The listing builds one solid part. Answer for the finished solid, in the listing's coordinates (mm). Round coordinates to 2 decimals unless told otherwise and drop trailing zeros. Loops run counter-clockwise (first coordinate to the right, second up) from the corner with the lowest first, then second, coordinate; pieces in that order, holes last. Notation, with made-up numbers: (-14, 68) -> (35, 68) arc R22 cw to (35, 77) -> close; hole circle Ø10 at (44, 8). An arc over 180 degrees is marked (long way). Use a Markdown table: item, result. Add a question column.
Q1. Given pin 1 Ø1 at (x, z) = (-13.73, -10.14) entering from -Y, flat-ended and moving along its own axis, determine where the tip first touches the part or whether it passes through.
Q2. Section A-A on y = 1 is taken. Give the number of separate pieces and of enclosed holes in the cut face, then the cut area to 3 significant figures.
Q3. Section B-B on z = 9 is taken. Give the vertices of the cut face in (x, y) (3 decimals).
Q4. Consider line 1 (Z direction, x = 7, y = 0.8) (3 decimals); line 2 (Z direction, x = 6.5, y = 0.7) (3 decimals). Determine where each line is inside the solid, lowest interval first.
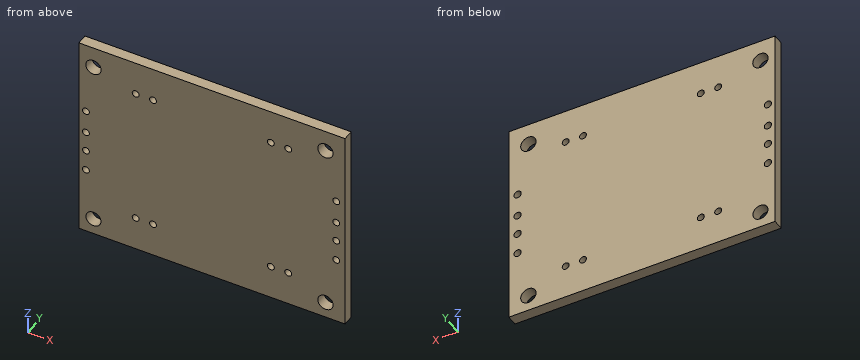
from build123d import *

# Parameters (mm, degrees)
SKETCH_1_W               = 30.85
SKETCH_1_H               = 24.07
EXTRUDE_1_DEPTH          = 1.25
CUT_EXTRUDE_1_DEPTH      = 11
CUT_EXTRUDE_1_DEPTH_BACK = 11
SKETCH_2_R               = 0.872176239
SKETCH_2_R_2             = 0.89
SKETCH_2_R_3             = 0.4


# Read off the part's stored shape, not the designer's step: 切除-拉伸2
with BuildPart() as part:
    # 草图1 → 凸台-拉伸1 (new body)
    with BuildSketch(Plane(origin=(0, 0, 0), x_dir=(1, 0, 0), z_dir=(0, 1, 0))):
        Rectangle(SKETCH_1_W, SKETCH_1_H)
    extrude(amount=EXTRUDE_1_DEPTH)

    # 草图2 → 切除-拉伸1 (cut, two sides: drawn at the far end of the back side and taken through both)
    with BuildSketch(Plane(origin=(0, 0, 0), x_dir=(1, 0, 0), z_dir=(0, 1, 0)).offset(-CUT_EXTRUDE_1_DEPTH_BACK)):
        with Locations(Location((-13.728729398, 10.145, 0), (0, 0, 270))):
            Circle(SKETCH_2_R)
        with Locations(Location((-13.728729398, -9.533026001, 0), (0, 0, 270))):
            Circle(SKETCH_2_R_2)
        with Locations(Location((13.15647485, -9.533026001, 0), (0, 0, 270))):
            Circle(SKETCH_2_R_2)
        with Locations(Location((13.15647485, 10.145, 0), (0, 0, 270))):
            Circle(SKETCH_2_R_2)
        with Locations(Location((-8.835, 8.055, 0), (0, 0, 270))):
            Circle(SKETCH_2_R_3)
        with Locations(Location((-6.825, 8.055, 0), (0, 0, 270))):
            Circle(SKETCH_2_R_3)
        with Locations(Location((6.825, 8.055, 0), (0, 0, 270))):
            Circle(SKETCH_2_R_3)
        with Locations(Location((8.835, 8.055, 0), (0, 0, 270))):
            Circle(SKETCH_2_R_3)
        with Locations(Location((-8.835, -8.055, 0), (0, 0, 270))):
            Circle(SKETCH_2_R_3)
        with Locations(Location((-6.825, -8.055, 0), (0, 0, 270))):
            Circle(SKETCH_2_R_3)
        with Locations(Location((6.825, -8.055, 0), (0, 0, 270))):
            Circle(SKETCH_2_R_3)
        with Locations(Location((8.835, -8.055, 0), (0, 0, 270))):
            Circle(SKETCH_2_R_3)
    extrude(amount=CUT_EXTRUDE_1_DEPTH + CUT_EXTRUDE_1_DEPTH_BACK, mode=Mode.SUBTRACT)

    # 切除-拉伸2 outline → 切除-拉伸2 (revolve, cut)
    with BuildSketch(Plane(origin=(14.403562721, 0, -4.132088396), x_dir=(1, 0, 0), z_dir=(0, 0, 1))):
        Polygon((0.421818831, 1.25), (0, 1.25), (0, 0), (0.4, 0), align=None)
    revolve(axis=Axis((14.403562721, 0, -4.132088396), (0, 1, 0)), mode=Mode.SUBTRACT)

    # Cut-Extrude 2 2 outline → Cut-Extrude 2 2 (revolve, cut)
    with BuildSketch(Plane(origin=(-14.599926989, 0, -4.132088396), x_dir=(1, 0, 0), z_dir=(0, 0, 1))):
        Polygon((0.421818831, 1.25), (0, 1.25), (0, 0), (0.4, 0), align=None)
    revolve(axis=Axis((-14.599926989, 0, -4.132088396), (0, 1, 0)), mode=Mode.SUBTRACT)

    # Cut-Extrude 2 3 outline → Cut-Extrude 2 3 (revolve, cut)
    with BuildSketch(Plane(origin=(14.403562721, 0, -1.635099216), x_dir=(1, 0, 0), z_dir=(0, 0, 1))):
        Polygon((0.421818831, 1.25), (0, 1.25), (0, 0), (0.4, 0), align=None)
    revolve(axis=Axis((14.403562721, 0, -1.635099216), (0, 1, 0)), mode=Mode.SUBTRACT)

    # Cut-Extrude 2 4 outline → Cut-Extrude 2 4 (revolve, cut)
    with BuildSketch(Plane(origin=(14.403562721, 0, 0.733839237), x_dir=(1, 0, 0), z_dir=(0, 0, 1))):
        Polygon((0.421818831, 1.25), (0, 1.25), (0, 0), (0.4, 0), align=None)
    revolve(axis=Axis((14.403562721, 0, 0.733839237), (0, 1, 0)), mode=Mode.SUBTRACT)

    # Cut-Extrude 2 5 outline → Cut-Extrude 2 5 (revolve, cut)
    with BuildSketch(Plane(origin=(14.403562721, 0, 3.486929872), x_dir=(1, 0, 0), z_dir=(0, 0, 1))):
        Polygon((0.421818831, 1.25), (0, 1.25), (0, 0), (0.4, 0), align=None)
    revolve(axis=Axis((14.403562721, 0, 3.486929872), (0, 1, 0)), mode=Mode.SUBTRACT)

    # Cut-Extrude 2 6 outline → Cut-Extrude 2 6 (revolve, cut)
    with BuildSketch(Plane(origin=(-14.599926989, 0, 3.486929872), x_dir=(1, 0, 0), z_dir=(0, 0, 1))):
        Polygon((0.421818831, 1.25), (0, 1.25), (0, 0), (0.4, 0), align=None)
    revolve(axis=Axis((-14.599926989, 0, 3.486929872), (0, 1, 0)), mode=Mode.SUBTRACT)

    # Cut-Extrude 2 7 outline → Cut-Extrude 2 7 (revolve, cut)
    with BuildSketch(Plane(origin=(-14.599926989, 0, 0.733839237), x_dir=(1, 0, 0), z_dir=(0, 0, 1))):
        Polygon((0.421818831, 1.25), (0, 1.25), (0, 0), (0.4, 0), align=None)
    revolve(axis=Axis((-14.599926989, 0, 0.733839237), (0, 1, 0)), mode=Mode.SUBTRACT)

    # Cut-Extrude 2 8 outline → Cut-Extrude 2 8 (revolve, cut)
    with BuildSketch(Plane(origin=(-14.599926989, 0, -1.635099216), x_dir=(1, 0, 0), z_dir=(0, 0, 1))):
        Polygon((0.421818831, 1.25), (0, 1.25), (0, 0), (0.4, 0), align=None)
    revolve(axis=Axis((-14.599926989, 0, -1.635099216), (0, 1, 0)), mode=Mode.SUBTRACT)


solid = part.part
Checked values:
| question | item | result |
|---|---|---|
| 1 | pin 1 | passes through |
| 2 | separate pieces | 1 |
| 2 | enclosed holes | 20 |
| 2 | area | 724 mm2 |
| 3 | outline | (-15.425, 0) -> (-14.441, 0) -> (-14.441, 1.25) -> (-15.425, 1.25) -> close; (-13.016, 0) -> (12.444, 0) -> (12.444, 1.25) -> (-13.016, 1.25) -> close; (13.869, 0) -> (15.425, 0) -> (15.425, 1.25) -> (13.869, 1.25) -> close |
| 4 | line 1 | z = -12.035 to -8.415, -7.695 to 7.695, 8.415 to 12.035 |
| 4 | line 2 | z = -12.035 to -8.288, -7.822 to 7.822, 8.288 to 12.035 |
